```python
from build123d import *

# Parameters (mm, degrees)
SKETCH_1_R               = 30
SKETCH_1_R_2             = 6
EXTRUDE_1_DEPTH          = 14.6
FILLET_2_R               = 5
SKETCH_3_R               = 1.5
CUT_EXTRUDE_1_DEPTH      = 15.6
PATTERN_CIRCULAR_2_COUNT = 6


with BuildPart() as part:
    # ｽｹｯﾁ1 → ﾎﾞｽ - 押し出し1 (new body)
    with BuildSketch(Plane.XY):
        Circle(SKETCH_1_R)
        Circle(SKETCH_1_R_2, mode=Mode.SUBTRACT)
    extrude(amount=EXTRUDE_1_DEPTH)

    # ﾌｨﾚｯﾄ2
    fillet_2_edges = [part.edges().sort_by_distance(p)[0] for p in [
        (-30, 0, 0),
        (-30, 0, 14.6),
    ]]
    fillet(fillet_2_edges, radius=FILLET_2_R)

    # ｽｹｯﾁ3 → ｶｯﾄ - 押し出し1 (cut, through all)
    with BuildSketch(Plane(origin=(0, 0, 0), x_dir=(-1, 0, 0), z_dir=(0, 0, -1))):
        with Locations((0, 10.5)):
            Circle(SKETCH_3_R)
    cut_extrude_1 = extrude(amount=-CUT_EXTRUDE_1_DEPTH, mode=Mode.SUBTRACT)

    # 円形ﾊﾟﾀｰﾝ2: ｶｯﾄ - 押し出し1 ×6 about axis
    pattern_circular_2_axis = Axis((0, 0, 0), (0, 0, 1))
    for i in range(1, PATTERN_CIRCULAR_2_COUNT):
        add(cut_extrude_1.rotate(pattern_circular_2_axis, i * 360 / PATTERN_CIRCULAR_2_COUNT), mode=Mode.SUBTRACT)


solid = part.part
```
Verification items for the finished model (mm, model axes). Round coordinates to 2 decimals unless told otherwise and drop trailing zeros. Write each loop counter-clockwise with the first axis right and the second up, starting at its lowest first coordinate (ties: lowest second). Pieces come first, ordered by that corner, then holes.
1. Section check C-C on z = 8. Enter the section's corners in (x, y), plus the area to 3 significant figures.
2. Scan lines: L1, parallel to Y at x = 0, z = 9; L2, parallel to Y at x = -1, z = 4.25; L3, parallel to X at y = 1, z = 9. Record each from-to range of solid material in increasing order.
3. Gauge pin test, flat ends, axial feed: P1, Ø2.5, axis at x = 9.09, y = -5.25, coming from the -Z side; P2, Ø1.5, axis at x = -17.5, z = 3, coming from the +Y side; P3, Ø5, axis at x = -16, z = 10, coming from the -Y side; P4, Ø4, axis at x = -9.09, y = 5.25, coming from the +Z side. Record the tip position at first contact, or that the pin passes through.
4. Draft check along X on faces 1 (the flat face through (5, -5, 0)), 2 (the cylindrical face through (0, -9, 7)), 3 (the cylindrical face through (-29.97, 1.32, 7.27)). Enter one of: +X half, -X half, draft (parallel to the pull), parting line (faces both ways), or undercut.
5. Section check A-A on x = 0. Enter the section's corners in (y, z), plus the area to 3 significant figures.
6. Section check B-B on y = 0. Enter the section's corners in (x, z).
Answer:
1. outline: circle Ø60 at (0, 0); hole circle Ø3 at (-9.09, -5.25); hole circle Ø3 at (-9.09, 5.25); hole circle Ø12 at (0, 0); hole circle Ø3 at (0, -10.5); hole circle Ø3 at (0, 10.5); hole circle Ø3 at (9.09, -5.25); hole circle Ø3 at (9.09, 5.25)
1. area: 2,670 mm2
2. L1: y = -30 to -12, -9 to -6, 6 to 9, 12 to 30
2. L2: y = -29.93 to -11.62, -9.38 to -5.92, 5.92 to 9.38, 11.62 to 29.93
2. L3: x = -29.98 to -5.92, 5.92 to 29.98
3. P1: passes through
3. P2: stops at y = 24.49
3. P3: stops at y = -26.78
3. P4: stops at z = 14.6
4. face 1: draft
4. face 2: undercut
4. face 3: parting line
5. outline: (-30, 5) arc R5 ccw to (-25, 0) - (-12, 0) - (-12, 14.6) - (-25, 14.6) arc R5 ccw to (-30, 9.6) - close; (-9, 0) - (-6, 0) - (-6, 14.6) - (-9, 14.6) - close; (6, 0) - (9, 0) - (9, 14.6) - (6, 14.6) - close; (12, 0) - (25, 0) arc R5 ccw to (30, 5) - (30, 9.6) arc R5 ccw to (25, 14.6) - (12, 14.6) - close
5. area: 592 mm2
6. outline: (-30, 5) arc R5 ccw to (-25, 0) - (-6, 0) - (-6, 14.6) - (-25, 14.6) arc R5 ccw to (-30, 9.6) - close; (6, 0) - (25, 0) arc R5 ccw to (30, 5) - (30, 9.6) arc R5 ccw to (25, 14.6) - (6, 14.6) - close
